from build123d import *

# Parameters (mm, degrees)
F0_R            = 125
F2_DEPTH        = 5
F1_R            = 15
F3_DEPTH        = 5.001
F5_D            = 5
F5_COPIES_COUNT = 4


# Not quite as in the source:
# - a pattern or mirror of a feature is missing from the dataset's text; its kind, count and spacing are read off the source's solid
# - a feature names something its author has since deleted; it is built from what else it names


with BuildPart() as f2:
    # F0 (on Top) → F2 (new body)
    with BuildSketch(Plane.XY):
        Circle(F0_R)
    extrude(amount=F2_DEPTH)

    # F1 (on Top) → F3 (cut, through all)
    with BuildSketch(Plane.XY):
        Circle(F1_R)
    extrude(amount=F3_DEPTH, mode=Mode.SUBTRACT)

    # F5 (through all)
    with Locations(Plane(origin=(0, 0, 0), x_dir=(1, 0, 0), z_dir=(0, 0, -1))):
        with Locations((0, -27)):
            f5 = Hole(F5_D / 2)

    # F5_copies: F5 ×4 about axis
    f5_copies_axis = Axis((0, 0, 0), (0, 0, 1))
    for i in range(1, F5_COPIES_COUNT):
        add(f5.rotate(f5_copies_axis, i * 360 / F5_COPIES_COUNT), mode=Mode.SUBTRACT)


solid = f2.part
Check sheet for the modelled part. Datum: model origin and axes. Units: mm. Give positions to 0.01 mm unless a question says otherwise; leave off trailing zeros. Order: outer loops, then holes, each group sorted by start corner. A loop starts at its lowest first (then second) coordinate and runs counter-clockwise, first axis right, second up. Notation, with made-up numbers: M 53,-17 L 100,-17 A18 ccw 100,-5 Z; hole C 46,-21 d6. An arc over 180 degrees is marked long. Answer as CSV lines item,"result". Start each with the question number.
Item 1: Thickness scan on line 1 (Y direction, x = 0, z = 2.1); line 2 (Y direction, x = 2, z = 0.8); line 3 (Y direction, x = 27, z = 2.6). Record the ranges inside material, lowest first. Write a range as [from, to].
Item 2: Cross-section at C-C on y = 51. Enter the section's corners in (x, z).
Item 3: Cross-section at A-A on y = -7. Enter the section's corners in (x, z), plus the area to 3 significant figures.
Item 4: Mould release check, pull along Y, two halves, no side actions. Record for faces 1 (the face through (-14.985, 0.66, 2.465)), 2 (the face through (-124.88, 5.5, 2.46)), 3 (the face through (-30, 2, 5)): +Y half, -Y half, draft (parallel to the pull), parting line (faces both ways), or undercut.
Item 5: Gauge pin test, flat ends, axial feed: P1, Ø4.5, axis at x = 27, y = 0, coming from the +Z side; P2, Ø6, axis at x = 0, y = -27, coming from the +Z side; P3, Ø2, axis at x = -59.5, z = 2.5, coming from the -Y side; P4, Ø1, axis at y = 80.5, z = 2, coming from the +X side. Record the tip position at first contact, or that the pin passes through.
Item 6: Cross-section at D-D on x = 49. Enter the section's corners in (y, z), plus the area to 3 significant figures.
Item 7: Cross-section at B-B on z = 1. Enter the section's corners in (x, y), plus the area to 3 significant figures.
Established:
1,line 1,"y = [-125, -29.5], [-24.5, -15], [15, 24.5], [29.5, 125]"
1,line 2,"y = [-124.98, -28.5], [-25.5, -14.87], [14.87, 25.5], [28.5, 124.98]"
1,line 3,"y = [-122.05, -2.5], [2.5, 122.05]"
2,outline,"M -114.12,0 L 114.12,0 L 114.12,5 L -114.12,5 Z"
3,outline,"M -124.8,0 L -13.27,0 L -13.27,5 L -124.8,5 Z; M 13.27,0 L 124.8,0 L 124.8,5 L 13.27,5 Z"
3,area,"1,120 mm^2"
4,face 1,"undercut"
4,face 2,"parting line"
4,face 3,"draft"
5,P1,"passes through"
5,P2,"stops at z = 5"
5,P3,"stops at y = -110.47"
5,P4,"stops at x = 96.05"
6,outline,"M -115,0 L 115,0 L 115,5 L -115,5 Z"
6,area,"1,150 mm^2"
7,outline,"C 0,0 d250; hole C -27,0 d5; hole C 0,0 d30; hole C 0,-27 d5; hole C 0,27 d5; hole C 27,0 d5"
7,area,"48,300 mm^2"
